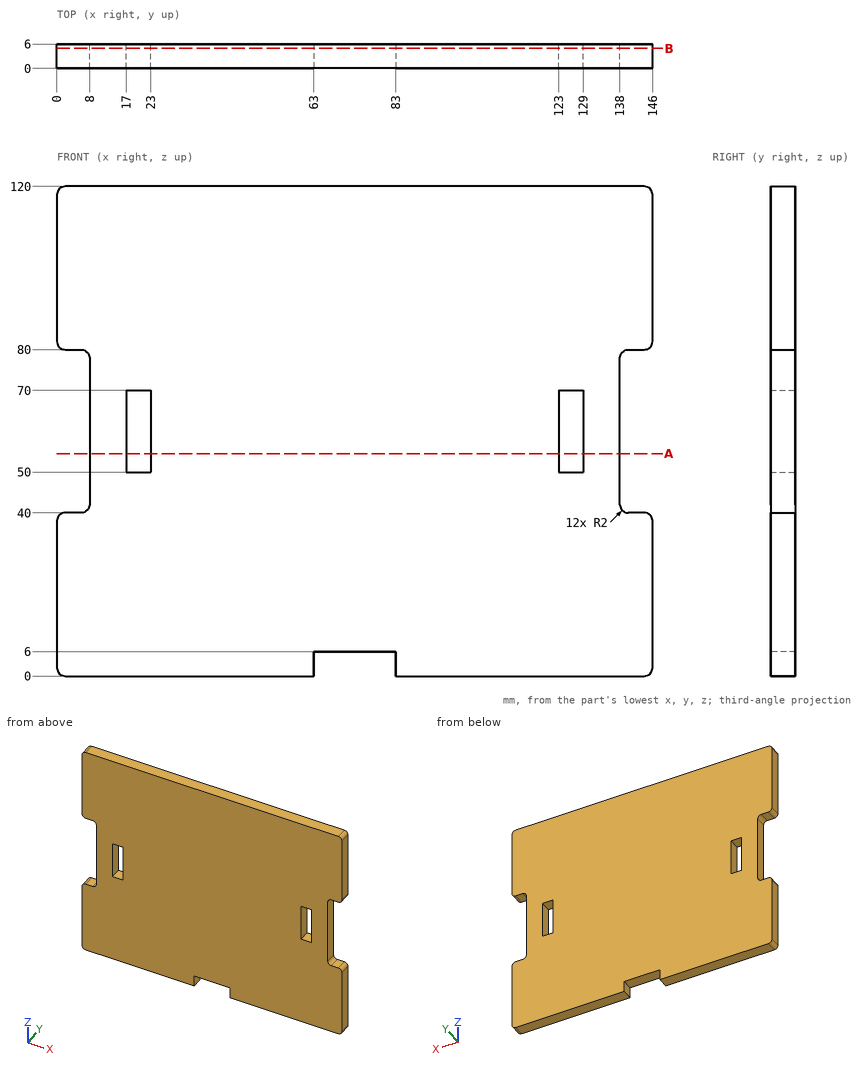
Drawing for the job (mm, zero at the part's lowest x, y, z). Give positions to 0.01 mm unless a question says otherwise; leave off trailing zeros. Loops run counter-clockwise (first coordinate to the right, second up) from the corner with the lowest first, then second, coordinate; pieces in that order, holes last.
Item 1: Drill centre lines: line 1 along X through (y, z) = (0.7, 59); line 2 along Z through (x, y) = (18, 4.35); line 3 along Z through (x, y) = (75, 4.7). Where is each one in solid material? Low to high.
Check values:
line 1: x = 8 to 17, 23 to 123, 129 to 138
line 2: z = 0 to 50, 70 to 120
line 3: z = 6 to 120
Item 2: Slice it at B-B (y = 4.9). Give the number of separate pieces and of enclosed holes in the cut face, plus the area to 3 significant figures.
Check values:
separate pieces: 1
enclosed holes: 2
area: 16,500 mm2
Item 3: Slice it at A-A (z = 54.5). Write the cut outline in (x, y).
Check values:
outline: (8, 0) - (17, 0) - (17, 6) - (8, 6) - close; (23, 0) - (123, 0) - (123, 6) - (23, 6) - close; (129, 0) - (138, 0) - (138, 6) - (129, 6) - close
Item 4: Drop flat-ended pins along their axis: P1, Ø3, axis at x = 77, y = 4.5, coming from the -Z side; P2, Ø1.8, axis at y = 1.5, z = 55.5, coming from the -X side; P3, Ø1.8, axis at y = 2.5, z = 64.5, coming from the +X side. Give the stop position or say it passes through.
Check values:
P1: stops at z = 6
P2: stops at x = 8
P3: stops at x = 138
